Autodesk Inventor part; units mm, degrees
ref_plane "YZ Plane" through (0, 0, 0) normal (1, 0, 0) x (0, 1, 0)
ref_plane "XZ Plane" through (0, 0, 0) normal (0, 1, 0) x (-1, 0, 0)
ref_plane "XY Plane" through (0, 0, 0) normal (0, 0, 1) x (1, 0, 0)
sketch "Sketch1" plane through (0, 0, 0) normal (0, 0, 1) x (1, 0, 0)
  line L0 (0, 0) -> (58, 0)
  line L1 (58, 0) -> (58, 138)
  line L2 (58, 138) -> (0, 138)
  line L3 (0, 138) -> (0, 0)
  dimension "d0" = 58
  dimension "d1" = 138
extrude "Extrusion1" add sketch "Sketch1" along normal blind 5
sketch "Sketch2" plane through (0, 0, 5) normal (0, 0, 1) x (1, 0, 0)
  circle A0 centre (53, 5) radius 1.5
  circle A1 centre (5.8194, 5) radius 1.5
  line L0 (58, 138) -> (0, 138)
  line L1 (0, 138) -> (0, 0)
  circle A2 centre (5.4959, 133) radius 1.5
  line L2 (58, 0) -> (58, 138)
  circle A3 centre (53, 133) radius 1.5
  dimension "d6" = 3
  dimension "d8" = 3
  dimension "d10" = 3
  dimension "d13" = 3
extrude "Extrusion2" cut sketch "Sketch2" against normal through all
fillet "Fillet1" radius 2 2 edges at (58, 69, 5) (0, 69, 5)
sketch "Sketch3" plane through (0, 0, 5) normal (0, 0, 1) x (1, 0, 0)
  line L0 (56, 138) -> (2, 138)
  circle A0 centre (29, 88) radius 6.5
  line L1 (0, 0) -> (58, 0)
  circle A1 centre (29, 50) radius 6.5
  dimension "d18" = 13
  dimension "d20" = 13
extrude "Extrusion3" cut sketch "Sketch3" against normal through all
properties part number "ICE CREAM COVER"
Build history of the part. All positions in model axes, mm. Round coordinates to 2 decimals unless told otherwise and drop trailing zeros. Loops run counter-clockwise (first coordinate to the right, second up) from the corner with the lowest first, then second, coordinate; pieces in that order, holes last.
Item 1: Saw through at B-B (y = 133). List the corners of the cut face in (x, z).
Item 2: Drill centre lines: line 1 along Y through (x, z) = (29, 2.8); line 2 along Y through (x, z) = (53, 3.8); line 3 along X through (y, z) = (92.5, 4.65). Where is each one in solid material? Low to high.
Item 3: Saw through at D-D (z = 2.2). List the corners of the cut face in (x, y).
Item 4: Saw through at A-A (x = 29). List the corners of the cut face in (y, z), then the cut area to 3 significant figures.
Item 5: Saw through at C-C (y = 88). List the corners of the cut face in (x, z), then the cut area to 3 significant figures.
Item 6: Two-plate mould, pull along Y, no slides. Class faces 1 (the face through (27.591, 43.655, 2.535)), 2 (the face through (29, 138, 2)), 3 (the face through (58, 68, 1)), 4 (the face through (5.301, 134.487, 2.535)): released by +Y, released by -Y, zero draft, split by the parting line, or undercut.
Worked answers:
1. outline: (0, 0) - (4, 0) - (4, 5) - (2, 5) arc R2 ccw to (0, 3) - close; (7, 0) - (51.5, 0) - (51.5, 5) - (7, 5) - close; (54.5, 0) - (58, 0) - (58, 3) arc R2 ccw to (56, 5) - (54.5, 5) - close
2. line 1: y = 0 to 43.5, 56.5 to 81.5, 94.5 to 138
2. line 2: y = 0 to 3.5, 6.5 to 131.5, 134.5 to 138
2. line 3: x = 0.87 to 24.31, 33.69 to 57.13
3. outline: (0, 0) - (58, 0) - (58, 138) - (0, 138) - close; hole circle Ø3 at (5.5, 133); hole circle Ø3 at (5.82, 5); hole circle Ø13 at (29, 50); hole circle Ø13 at (29, 88); hole circle Ø3 at (53, 5); hole circle Ø3 at (53, 133)
4. outline: (0, 0) - (43.5, 0) - (43.5, 5) - (0, 5) - close; (56.5, 0) - (81.5, 0) - (81.5, 5) - (56.5, 5) - close; (94.5, 0) - (138, 0) - (138, 5) - (94.5, 5) - close
4. area: 560 mm2
5. outline: (0, 0) - (22.5, 0) - (22.5, 5) - (2, 5) arc R2 ccw to (0, 3) - close; (35.5, 0) - (58, 0) - (58, 3) arc R2 ccw to (56, 5) - (35.5, 5) - close
5. area: 223 mm2
6. face 1: undercut
6. face 2: released by +Y
6. face 3: zero draft
6. face 4: undercut
